Geometry check sheet. Reference: the model listing, model coordinates, mm. Face numbers are marked on the shaded views. A direction names the side the tool comes from. Round coordinates to 2 decimals unless told otherwise and drop trailing zeros. Write each loop counter-clockwise with the first axis right and the second up, starting at its lowest first coordinate (ties: lowest second). Pieces come first, ordered by that corner, then holes.
Item 1: Scan lines: probe 1 along Y at (x, z) = (19, 15.5); probe 2 along X at (y, z) = (-2.5, 33); probe 3 along X at (y, z) = (-0.5, 49). Record each from-to range of solid material in increasing order.
Item 2: Access from +Z, -Z, +X, -X, +Y, -Y to the whole of each face (thin tool, end or side, straight path). Record for the marked faces 1, 2 and 3.
Item 3: Cross-section at D-D (y = -5.5). Enter the section's corners in (x, z), then the cut area to 3 significant figures.
Item 4: Depth check by flat-ended pin: P1, Ø2, axis at x = 4.5, y = -7, coming from the +Z side; P2, Ø3.5, axis at y = -3, z = 29.5, coming from the +X side; P3, Ø0.8, axis at x = 5, y = -0.5, coming from the -Z side. Enter the tip coordinate at first touch or a pass-through.
Item 5: Cross-section at B-B (x = 13). Enter the section's corners in (y, z).
Item 6: Cross-section at A-A (z = 22.5). Enter the section's corners in (x, y).
Item 7: Cross-section at C-C (z = 44). Enter the section's corners in (x, y).
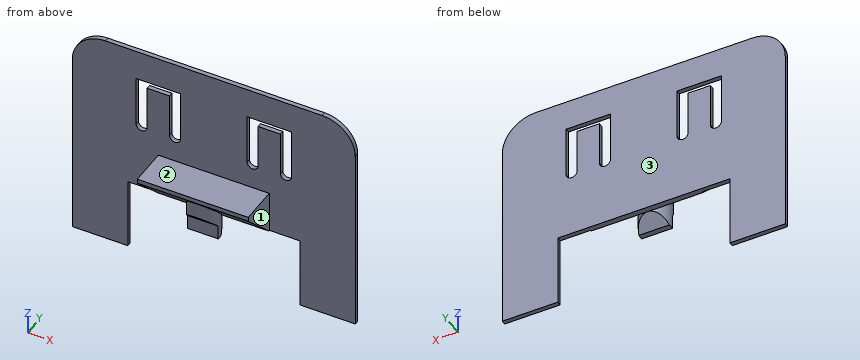
from build123d import *

# Parameters (mm, degrees)
PAD_DEPTH       = 0.8
PAD001_DEPTH    = 10
SKETCH003_R     = 2.8
PAD002_DEPTH    = 9.5
POCKET001_DEPTH = 3
POCKET_DEPTH    = 5


with BuildPart() as part:
    # Sketch → Pad (new body)
    with BuildSketch(Plane.XZ):
        with BuildLine():
            Line((-25.5, 13.5), (-25.5, 47.5))
            ThreePointArc((-19.5, 53.5), (-23.742641, 51.742641), (-25.5, 47.5))
            Line((-19.5, 53.5), (19.5, 53.5))
            ThreePointArc((25.5, 47.5), (23.742641, 51.742641), (19.5, 53.5))
            Line((25.5, 47.5), (25.5, 13.5))
            Line((25.5, 13.5), (15.5, 13.5))
            Line((15.5, 13.5), (15.5, 26.5))
            Line((15.5, 26.5), (-15.5, 26.5))
            Line((-15.5, 26.5), (-15.5, 13.5))
            Line((-15.5, 13.5), (-25.5, 13.5))
        make_face()
    extrude(amount=PAD_DEPTH)

    # Sketch001 → Pad001 (join, symmetric)
    with BuildSketch(Plane.YZ):
        Polygon((-1, 26.5), (-7.7, 33.2), (-7.7, 34), (0, 34), (0, 26.5), align=None)
    extrude(amount=PAD001_DEPTH, both=True)

    # Sketch003 (on Face12 of Pad001) → Pad002 (join)
    with BuildSketch(Plane(origin=(0, 0, 34), x_dir=(-1, 0, 0), z_dir=(0, 0, 1))):
        with Locations((0, 4)):
            Circle(SKETCH003_R)
    extrude(amount=-PAD002_DEPTH)

    # Sketch004 → Pocket001 (cut, symmetric)
    with BuildSketch(Plane.YZ):
        Polygon((-1.2, 26.699), (-3.399, 24.5), (-1.2, 24.5), align=None)
        Polygon((-7.7, 30.4), (-7.7, 24.5), (-4.4, 24.5), (-4.4, 27.1), align=None)
    extrude(amount=POCKET001_DEPTH, both=True, mode=Mode.SUBTRACT)

    # Sketch005 (on Face5 of Pad002) → Pocket (cut)
    with BuildSketch(Plane.XZ.offset(0.8)):
        with BuildLine():
            Line((-12, 38.8), (-12, 46.8))
            Line((-12, 46.8), (-8, 46.8))
            Line((-8, 46.8), (-8, 38.8))
            ThreePointArc((-8, 38.8), (-7, 37.8), (-6, 38.8))
            Line((-6, 38.8), (-6, 48))
            Line((-6, 48), (-14, 48))
            Line((-14, 48), (-14, 38.8))
            ThreePointArc((-14, 38.8), (-13, 37.8), (-12, 38.8))
        make_face()
        with BuildLine():
            Line((12, 38.8), (12, 46.8))
            Line((12, 46.8), (8, 46.8))
            Line((8, 46.8), (8, 38.8))
            ThreePointArc((6, 38.8), (7, 37.8), (8, 38.8))
            Line((6, 38.8), (6, 48))
            Line((6, 48), (14, 48))
            Line((14, 48), (14, 38.8))
            ThreePointArc((12, 38.8), (13, 37.8), (14, 38.8))
        make_face()
    extrude(amount=-POCKET_DEPTH, mode=Mode.SUBTRACT)


solid = part.part
Resolved:
1. probe 1: y = -0.8 to 0
1. probe 2: x = -10 to 10
1. probe 3: x = -25.31 to 25.31
2. face 1: +Z, -Z, +X, -Y
2. face 2: +Z, +X, -X, -Y
2. face 3: +Z, -Z, +X, -X, +Y
3. outline: (-10, 31) - (-2.36, 31) - (-2.36, 28.2) - (2.36, 28.2) - (2.36, 31) - (10, 31) - (10, 34) - (-10, 34) - close
3. area: 73.2 mm2
4. P1: stops at z = 34
4. P2: stops at x = 10
4. P3: stops at z = 26.5
5. outline: (-0.8, 26.5) - (0, 26.5) - (0, 37.8) - (-0.8, 37.8) - close; (-0.8, 48) - (0, 48) - (0, 53.5) - (-0.8, 53.5) - close
6. outline: (-25.5, -0.8) - (-15.5, -0.8) - (-15.5, 0) - (-25.5, 0) - close; (15.5, -0.8) - (25.5, -0.8) - (25.5, 0) - (15.5, 0) - close
7. outline: (-25.5, -0.8) - (-14, -0.8) - (-14, 0) - (-25.5, 0) - close; (-12, -0.8) - (-8, -0.8) - (-8, 0) - (-12, 0) - close; (-6, -0.8) - (6, -0.8) - (6, 0) - (-6, 0) - close; (8, -0.8) - (12, -0.8) - (12, 0) - (8, 0) - close; (14, -0.8) - (25.5, -0.8) - (25.5, 0) - (14, 0) - close
